Verification items for the finished model (mm, model axes). A direction names the side the tool comes from. Round coordinates to 2 decimals unless told otherwise and drop trailing zeros. Write each loop counter-clockwise with the first axis right and the second up, starting at its lowest first coordinate (ties: lowest second). Pieces come first, ordered by that corner, then holes.
from build123d import *

# Parameters (mm, degrees)
SKETCH1_W               = 31.75
SKETCH1_H               = 31.75
SKETCH1_W_2             = 25.654
SKETCH1_H_2             = 25.654
BOSS_EXTRUDE1_DEPTH     = 152.4
CUT_EXTRUDE1_DEPTH      = 16.875
CUT_EXTRUDE1_DEPTH_BACK = 16.875


with BuildPart() as part:
    # Sketch1 → Boss-Extrude1 (new body)
    with BuildSketch(Plane.XY):
        Rectangle(SKETCH1_W, SKETCH1_H)
        Rectangle(SKETCH1_W_2, SKETCH1_H_2, mode=Mode.SUBTRACT)
    extrude(amount=BOSS_EXTRUDE1_DEPTH)

    # Sketch2 → Cut-Extrude1 (cut, two sides)
    with BuildSketch(Plane(origin=(0, 0, 0), x_dir=(0, 0, -1), z_dir=(1, 0, 0))) as cut_extrude1_sk:
        Polygon((-152.4, 15.875), (-113.19201528, -15.875), (-152.4, -15.875), align=None)
    extrude(amount=CUT_EXTRUDE1_DEPTH, mode=Mode.SUBTRACT)
    extrude(cut_extrude1_sk.sketch, amount=-CUT_EXTRUDE1_DEPTH_BACK, mode=Mode.SUBTRACT)


solid = part.part
Q1. Sectioned sample at B-B (x = 6.5). Enter the section's corners in (y, z) (3 decimals).
Recorded:
outline: (-15.875, 0) - (-12.827, 0) - (-12.827, 116.956) - (-15.875, 113.192) - close; (12.827, 0) - (15.875, 0) - (15.875, 152.4) - (12.827, 148.636) - close
Q2. Sectioned sample at A-A (z = 44). Enter the section's corners in (x, y) (3 decimals).
Recorded:
outline: (-15.875, -15.875) - (15.875, -15.875) - (15.875, 15.875) - (-15.875, 15.875) - close; hole (-12.827, -12.827) - (12.827, -12.827) - (12.827, 12.827) - (-12.827, 12.827) - close
Q3. Release check for a two-part mould opening along X. For faces 1 (the flat face through (0, -15.875, 56)), 2 (the flat face through (-15.875, 0, 58)), 3 (the flat face through (0, -12.827, 58)), 4 (the flat face through (12.827, 0, 73)) record: released by +X, released by -X, zero draft, split by the parting line, or undercut.
Recorded:
face 1: zero draft
face 2: released by -X
face 3: undercut
face 4: undercut
Q4. Material ranges on line 1 along Y through (x, z) = (1, 46) (3 decimals); line 2 along Y through (x, z) = (8.5, 141.5) (3 decimals), recorded low to high.
Recorded:
line 1: y = -15.875 to -12.827, 12.827 to 15.875
line 2: y = 12.827 to 15.875
Q5. Tool access check on faces 5 (the flat face through (0, 12.827, 73)), 6 (the flat face through (15.875, 0, 58)). Record the directions out of +Z, -Z, +X, -X, +Y, -Y that give a thin tool (end or side, any length) a straight path to the whole face; none if there is none.
Recorded:
face 5: +Z, -Z
face 6: +Z, -Z, +X, +Y, -Y
Q6. Depth check by flat-ended pin: P1, Ø6, axis at x = -1, y = 10.5, coming from the -Z side. Enter the tip coordinate at first touch or a pass-through.
Recorded:
P1: stops at z = 0
Q7. Sectioned sample at C-C (y = 2.5). Enter the section's corners in (x, z) (3 decimals), plus the area to 3 significant figures.
Recorded:
outline: (-15.875, 0) - (-12.827, 0) - (-12.827, 135.883) - (-15.875, 135.883) - close; (12.827, 0) - (15.875, 0) - (15.875, 135.883) - (12.827, 135.883) - close
area: 828 mm2
